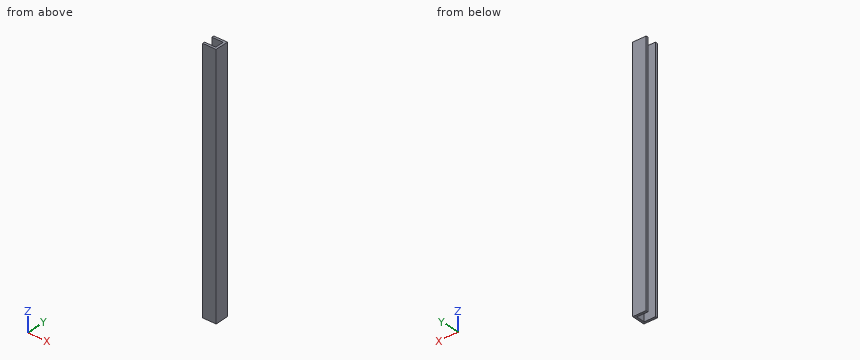
Autodesk Inventor part; units mm, degrees
ref_plane "YZ Plane" through (0, 0, 0) normal (1, 0, 0) x (0, 1, 0)
ref_plane "XZ Plane" through (0, 0, 0) normal (0, 1, 0) x (-1, 0, 0)
ref_plane "XY Plane" through (0, 0, 0) normal (0, 0, 1) x (1, 0, 0)
sketch "Sketch1" plane through (0, 0, 0) normal (0, 0, 1) x (1, 0, 0)
  line L0 (-16.8285, 19.5793) -> (2.2215, 19.5793)
  line L1 (2.2215, 19.5793) -> (2.2215, 0.5293)
  line L2 (2.2215, 0.5293) -> (-16.8285, 0.5293)
  line L3 (-16.8285, 0.5293) -> (-16.8285, 19.5793)
  line L4 (-16.8285, 16.4043) -> (-0.9535, 16.4043)
  line L5 (-0.9535, 16.4043) -> (-0.9535, 3.7043)
  line L6 (-0.9535, 3.7043) -> (-16.8285, 3.7043)
  line L7 (-16.8285, 3.7043) -> (-16.8285, 16.4043)
  dimension "d0" = 19.05
  dimension "d1" = 19.05
  dimension "d2" = 3.175
  dimension "d3" = 3.175
  dimension "d4" = 3.175
extrude "Extrusion1" add sketch "Sketch1" along normal blind 355.6 contours L0 L1 L2 L3 L6 L5 L4
properties part number "GE-12016-08"
Here's how the part is built. I have some questions about the finished solid (model axes, mm). Give positions to 0.01 mm unless a question says otherwise; leave off trailing zeros. Write each loop counter-clockwise with the first axis right and the second up, starting at its lowest first coordinate (ties: lowest second). Pieces come first, ordered by that corner, then holes. Notation, with made-up numbers: (50.5, 22) -> (90.5, 22) arc R33 ccw to (90.5, 54) -> close; hole circle Ø4 at (47, 15). An arc over 180 degrees is marked (long way). Use one line per item in the form item = value. Start each with the question number.
1. Imagine slicing it at B-B on z = 223. List the corners of the cut face in (x, y) for me.
2. Will these pins go through, and if not, where does the flat tip stop? pin 1 Ø8 at (y, z) = (6, 231.5) entering from -X; pin 2 Ø1.5 at (y, z) = (14, 134) entering from -X.
3. Imagine slicing it at C-C on y = 11.5. List the corners of the cut face in (x, z) for me.
4. If I drill on L1, parallel to Y at x = -4.25, z = 206; L2, parallel to X at y = 8, z = 34.5, over which ranges is the centre line in solid material (lowest first)?
5. Imagine slicing it at A-A on x = -5.5. List the corners of the cut face in (y, z) for me.
Entries:
q1.outline = (-16.83, 0.53) -> (2.22, 0.53) -> (2.22, 19.58) -> (-16.83, 19.58) -> (-16.83, 16.4) -> (-0.95, 16.4) -> (-0.95, 3.7) -> (-16.83, 3.7) -> close
q2.pin_1 = -16.83
q2.pin_2 = -0.95
q3.outline = (-0.95, 0) -> (2.22, 0) -> (2.22, 355.6) -> (-0.95, 355.6) -> close
q4.L1 = 0.53 to 3.7, 16.4 to 19.58
q4.L2 = -0.95 to 2.22
q5.outline = (0.53, 0) -> (3.7, 0) -> (3.7, 355.6) -> (0.53, 355.6) -> close; (16.4, 0) -> (19.58, 0) -> (19.58, 355.6) -> (16.4, 355.6) -> close
